Input: dimensioned drawing with shaded views. Units: mm. Origin: part minimum x, y, z. Round coordinates to 2 decimals unless told otherwise and drop trailing zeros. Loops run counter-clockwise (first coordinate to the right, second up) from the corner with the lowest first, then second, coordinate; pieces in that order, holes last. Notation, with made-up numbers: M 77.5,86 L 108.5,86 A26 cw 108.5,110 Z; hole C -8.5,63.25 d11. An arc over 180 degrees is marked long. Use one line per item in the form item = value. Start each with the question number.
Q1. Section query B-B, the plane z = 25. Output: boundary loops of the cut face in (x, y), and give its area (3 significant figures).
Q2. Section query A-A, the plane x = 26.5. Output: boundary loops of the cut face in (y, z).
Q3. First-contact query: P1, Ø6, axis at x = 33, z = 24, coming from the -Y side; P2, Ø17, axis at x = 20.5, z = 16, coming from the +Y side. Flat tips, straight axial feed; report the tip coordinate or a pass-through.
Q4. Section query C-C, the plane x = 22. Output: boundary loops of the cut face in (y, z).
Q5. Mould query, pull axis Z, two halves, no side actions, for the marked faces 1, 2, 3 and 4. Classes: pulls with the +Z half, pulls with the -Z half, needs draft (parallel to the pull), parting line crosses it, or undercut.
Q6. Ray query, line 1 along X through (y, z) = (2.45, 5); line 2 along X through (y, z) = (3.8, 25); line 3 along X through (y, z) = (3.85, 9.5). Return the intervals inside material, ascending.
Q7. Section query D-D, the plane y = 1.4. Output: boundary loops of the cut face in (x, z), and give its area (3 significant figures).
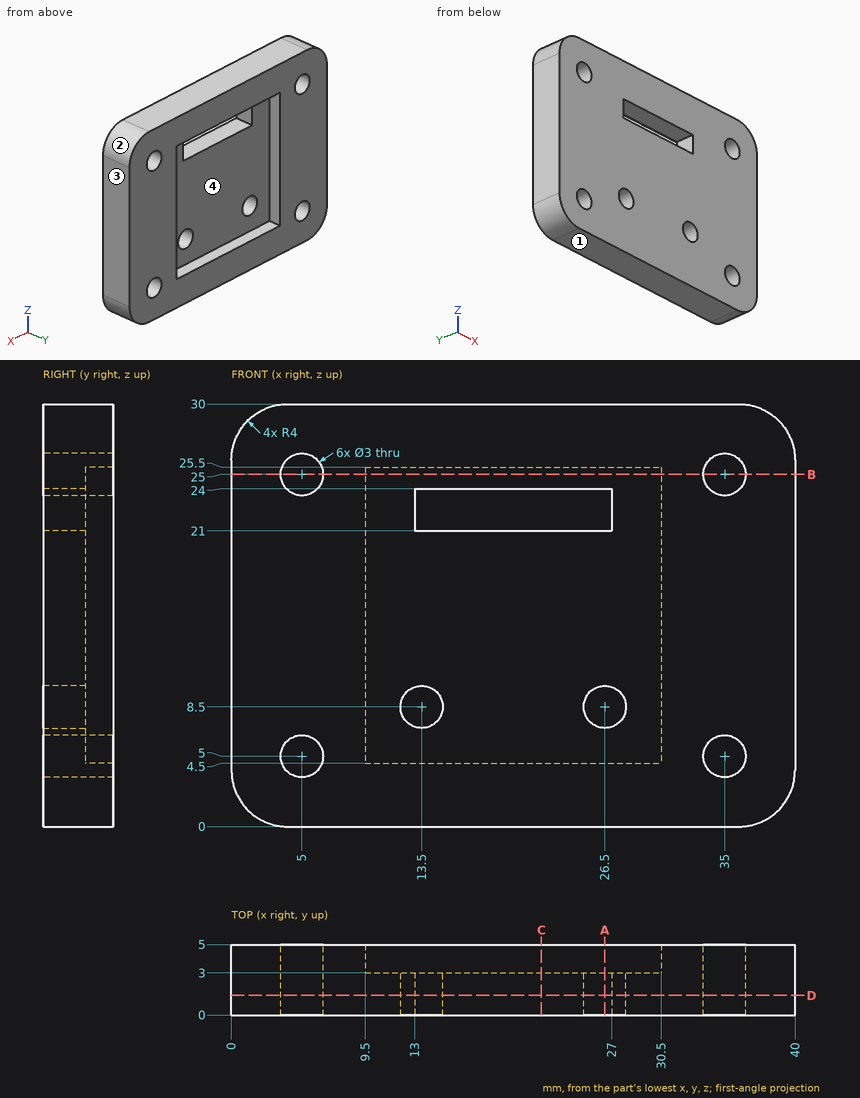
Results found:
q1.outline = M 0,0 L 3.5,0 L 3.5,5 L 0,5 Z; M 6.5,0 L 33.5,0 L 33.5,5 L 30.5,5 L 30.5,3 L 9.5,3 L 9.5,5 L 6.5,5 Z; M 36.5,0 L 40,0 L 40,5 L 36.5,5 Z
q1.area = 128 mm²
q2.outline = M 0,0 L 5,0 L 5,4.5 L 3,4.5 L 3,7 L 0,7 Z; M 0,10 L 3,10 L 3,21 L 0,21 Z; M 0,24 L 3,24 L 3,25.5 L 5,25.5 L 5,30 L 0,30 Z
q3.P1 = 0
q3.P2 = 3
q4.outline = M 0,0 L 5,0 L 5,4.5 L 3,4.5 L 3,21 L 0,21 Z; M 0,24 L 3,24 L 3,25.5 L 5,25.5 L 5,30 L 0,30 Z
q5.face_1 = pulls with the -Z half
q5.face_2 = pulls with the +Z half
q5.face_3 = needs draft
q5.face_4 = undercut
q6.line_1 = 0 to 3.5, 6.5 to 33.5, 36.5 to 40
q6.line_2 = 0 to 3.5, 6.5 to 9.5, 30.5 to 33.5, 36.5 to 40
q6.line_3 = 0 to 9.5, 30.5 to 40
q7.outline = M 0,4 A4 ccw 4,0 L 36,0 A4 ccw 40,4 L 40,26 A4 ccw 36,30 L 4,30 A4 ccw 0,26 Z; hole C 5,5 d3; hole C 5,25 d3; hole C 13.5,8.5 d3; hole M 13,21 L 27,21 L 27,24 L 13,24 Z; hole C 26.5,8.5 d3; hole C 35,5 d3; hole C 35,25 d3
q7.area = 1,100 mm²
